from build123d import *

# Parameters (mm, degrees)
SKETCH1_R           = 2.5
BOSS_EXTRUDE1_DEPTH = 57.2
SKETCH2_R           = 3.5
BOSS_EXTRUDE2_DEPTH = 2
CHAMFER1_SIZE       = 1
SKETCH3_R           = 1.5
CUT_EXTRUDE1_DEPTH  = 5


with BuildPart() as part:
    # Sketch1 → Boss-Extrude1 (new body)
    with BuildSketch(Plane(origin=(0, 0, 0), x_dir=(1, 0, 0), z_dir=(0, 1, 0))):
        Circle(SKETCH1_R)
    extrude(amount=BOSS_EXTRUDE1_DEPTH)

    # Sketch2 → Boss-Extrude2 (add)
    with BuildSketch(Plane(origin=(0, 57.2, 0), x_dir=(1, 0, 0), z_dir=(0, 1, 0))):
        Circle(SKETCH2_R)
    extrude(amount=BOSS_EXTRUDE2_DEPTH)

    # Chamfer1
    chamfer1_edges = [part.edges().sort_by_distance(p)[0] for p in [
        (-3.5, 59.2, 0),
    ]]
    chamfer(chamfer1_edges, length=CHAMFER1_SIZE)

    # Sketch3 → Cut-Extrude1 (cut)
    with BuildSketch(Plane.XZ):
        Circle(SKETCH3_R)
    extrude(amount=-CUT_EXTRUDE1_DEPTH, mode=Mode.SUBTRACT)


solid = part.part
Can you work these out from the model? Positions are in its coordinate system, mm. A direction names the side the tool comes from. Give positions to 0.01 mm unless a question says otherwise; leave off trailing zeros. Loops run counter-clockwise (first coordinate to the right, second up) from the corner with the lowest first, then second, coordinate; pieces in that order, holes last. Notation, with made-up numbers: (7, -30.5) -> (58, -30.5) arc R28 ccw to (58, -0.5) -> close; hole circle Ø6 at (75, 58). An arc over 180 degrees is marked (long way). Return JSON: item names as keys, results as strings.
Q1. I want a section at A-A, the plane z = 0. List the corners of the cut face in (x, y) for me, then the cut area to 3 significant figures.
Checks:
{"outline": "(-3.5, 57.2) -> (-2.5, 57.2) -> (-2.5, 0) -> (-1.5, 0) -> (-1.5, 5) -> (1.5, 5) -> (1.5, 0) -> (2.5, 0) -> (2.5, 57.2) -> (3.5, 57.2) -> (3.5, 58.2) -> (2.5, 59.2) -> (-2.5, 59.2) -> (-3.5, 58.2) -> close", "area": "284 mm2"}
Q2. I want a section at C-C, the plane y = 42. List the corners of the cut face in (x, z) for me.
Checks:
{"outline": "circle Ø5 at (0, 0)"}
Q3. I want a section at B-B, the plane x = 0. List the corners of the cut face in (y, z) for me, then the cut area to 3 significant figures.
Checks:
{"outline": "(0, -2.5) -> (57.2, -2.5) -> (57.2, -3.5) -> (58.2, -3.5) -> (59.2, -2.5) -> (59.2, 2.5) -> (58.2, 3.5) -> (57.2, 3.5) -> (57.2, 2.5) -> (0, 2.5) -> (0, 1.5) -> (5, 1.5) -> (5, -1.5) -> (0, -1.5) -> close", "area": "284 mm2"}
Q4. I need wall thicknesses on probe 1 along Z at (x, y) = (0, 2.55); probe 2 along X at (y, z) = (30, -0.25); probe 3 along X at (y, z) = (38, 2). Which ranges of each line are inside material? Lowest first, please.
Checks:
{"probe 1": "z = -2.5 to -1.5, 1.5 to 2.5", "probe 2": "x = -2.49 to 2.49", "probe 3": "x = -1.5 to 1.5"}
Q5. On a 3-axis mill with a long thin cutter (end or side, diameter ignored), from which of +Z, -Z, +X, -X, +Y, -Y can I reach the whole of each face in a straight line? I mean faces 4 (the face through (0, 5, 0)), 5 (the face through (0, 0, 2)). Say none if no direction works.
Checks:
{"face 4": "-Y", "face 5": "+Z, -Z, +X, -X, -Y"}
Q6. For pin 1 Ø3.5 at (x, z) = (0.5, 0) entering from -Y; pin 2 Ø4 at (y, z) = (37, 0.5) entering from +X; pin 3 Ø4 at (x, y) = (2, 43.5) entering from -Z; pin 4 Ø1.5 at (x, y) = (-1.5, 36.5) entering from +Z, each with a flat end and sliding along its axis, tell me the tip position at first contact or that it passes through.
Checks:
{"pin 1": "stops at y = 0", "pin 2": "stops at x = 2.5", "pin 3": "stops at z = -2.5", "pin 4": "stops at z = 2.38"}
Q7. We'd pull the mould along Z, two halves only. Please class faces 1 (the face through (-1.5, 2.46, 0.07)), 2 (the face through (3.233, 57.693, 1.341)), 3 (the face through (2, 57.2, 2)): released by +Z, released by -Z, zero draft, split by the parting line, or undercut.
Checks:
{"face 1": "undercut", "face 2": "split by the parting line", "face 3": "zero draft"}
